Part model, mm, in its own coordinate system. A direction names the side the tool comes from. Give positions to 0.01 mm unless a question says otherwise; leave off trailing zeros. Write each loop counter-clockwise with the first axis right and the second up, starting at its lowest first coordinate (ties: lowest second). Pieces come first, ordered by that corner, then holes.
from build123d import *

# Parameters (mm, degrees)
FILLET1_R           = 11
FILLET2_R           = 1
BOSS_EXTRUDE1_DEPTH = 10.425
CHAMFER1_SIZE       = 0.35


with BuildPart() as part:
    # Sketch1 → Revolve1 (revolve)
    with BuildSketch(Plane.XY, mode=Mode.PRIVATE) as revolve1_sk:
        with BuildLine():
            Line((0, 0), (8.5, 0))
            Line((8.5, 0), (8.5, 1))
            Line((8.5, 1), (6, 8))
            Line((6, 8), (6, 23))
            Line((6, 23), (5.5, 24))
            Line((5.5, 24), (4.5, 24))
            add(Edge.make_bspline(
                [(4.5, 24), (2.277777778, 23.5), (0, 23.5)],
                knots=[0, 0, 0, 1, 1, 1], degree=2))
            Line((0, 23.5), (0, 0))
        make_face()
    revolve(revolve1_sk.sketch.rotate(Axis((0, 23.5, 0), (0, -1, 0)), 180), axis=Axis((0, 23.5, 0), (0, -1, 0)))

    # Fillet1
    fillet1_edges = [part.edges().sort_by_distance(p)[0] for p in [
        (6, 8, 0),
    ]]
    fillet(fillet1_edges, radius=FILLET1_R)

    # Fillet2
    fillet2_edges = [part.edges().sort_by_distance(p)[0] for p in [
        (4.5, 24, 0),
        (5.5, 24, 0),
        (6, 23, 0),
        (8.5, 1, 0),
    ]]
    fillet(fillet2_edges, radius=FILLET2_R)

    # Sketch3 → Cut-Revolve1 (revolve, cut)
    with BuildSketch(Plane.XY, mode=Mode.PRIVATE) as cut_revolve1_sk:
        Polygon((0, 0), (3.875, 0), (3.875, 6.5), (3.05, 7.325), (3.05, 17.75), (0, 17.75), align=None)
    revolve(cut_revolve1_sk.sketch.rotate(Axis((0, 17.75, 0), (0, -1, 0)), 180), axis=Axis((0, 17.75, 0), (0, -1, 0)), mode=Mode.SUBTRACT)

    # Sketch4 → Boss-Extrude1 (add)
    with BuildSketch(Plane.XZ.offset(-17.75)):
        with BuildLine():
            Line((-2.655654345, 1.5), (2.655654345, 1.5))
            ThreePointArc((2.655654345, 1.5), (0, 3.05), (-2.655654345, 1.5))
        make_face()
        with BuildLine():
            ThreePointArc((-0.099986562, -3.048360656), (0, -3.05), (0.099986562, -3.048360656))
            ThreePointArc((0.099986562, -3.048360656), (0, -2.95), (-0.099986562, -3.048360656))
        make_face()
    extrude(amount=BOSS_EXTRUDE1_DEPTH)

    # Chamfer1
    # the kernel refuses this chamfer: 0.35 mm, written as the material it takes off along each edge
    with BuildSketch(Plane(origin=(-3.555743391, 7.325, 1.5), x_dir=(0, -0.02749587661058614, 0.9996219169112968), z_dir=(1, 0, 0))) as chamfer1_piece_1_section:
        Polygon((CHAMFER1_SIZE * 0.999621916911, -CHAMFER1_SIZE * 0.0274958766106), (-CHAMFER1_SIZE * 0.0274958766106, -CHAMFER1_SIZE * 0.999621916911), (0, 0), align=None)
    chamfer1_piece_1 = extrude(amount=7.111486782, mode=Mode.PRIVATE)
    chamfer1_piece_1 = chamfer1_piece_1 & Plane(origin=(0, 7.499624527, 0), x_dir=(-1, 0, 0), z_dir=(0, 1, 0)) * Cylinder(3.05, 16, mode=Mode.PRIVATE)
    add(chamfer1_piece_1, mode=Mode.SUBTRACT)


solid = part.part
1) Saw through at A-A (y = 18.5). Write the cut outline in (x, z).
Check result:
outline: circle Ø12 at (0, 0)
2) Drill centre lines: L1, parallel to Z at x = -0.25, y = 13.25; L2, parallel to Z at x = 2.25, y = 6.25; L3, parallel to Y at x = -3.5, z = 3.5. Where is each one in solid material? Low to high.
Check result:
L1: z = -5.99 to -3.04, 1.5 to 5.99
L2: z = -6.23 to -3.15, 3.15 to 6.23
L3: y = 0 to 24
3) Mould opens along X. For faces 1 (the cylindrical face through (-5.723, 16.425, -1.802)), 2 (the cylindrical face through (0.504, 3.296, -3.842)), 3 (the flat face through (4, 0, 2)) say: +X half, -X half, draft (parallel to the pull), parting line (faces both ways), or undercut.
Check result:
face 1: parting line
face 2: undercut
face 3: draft
4) Saw through at B-B (y = 4). Write the cut outline in (x, z) (3 decimals).
Check result:
outline: circle Ø14.857 at (0, 0); hole circle Ø7.75 at (0, 0)
5) 3-axis set-ups, long thin cutter, end or side, ignore diameter. For faces 4 (the flat face through (0, 7.325, 2)), 5 (the cylindrical face through (1.107, 0.419, -8.428)): which of +Z, -Z, +X, -X, +Y, -Y reach the whole face in a straight line?
Check result:
face 4: -Y
face 5: +Y, -Y
6) Flat gauge pins, fed straight in: P1, Ø3, axis at x = -3, z = 6.5, coming from the -Y side; P2, Ø2, axis at x = -4.5, y = 18, coming from the +Z side; P3, Ø10, axis at y = 13.5, z = -3, coming from the +X side; P4, Ø7, axis at x = 0, z = 0, coming from the -Y side (3 decimals). Where does each tip first touch, or does it go through?
Check result:
P1: stops at y = 0
P2: stops at z = 4.87
P3: stops at x = 6.01
P4: stops at y = 6.875
